The model under review builds one solid part; all positions refer to its coordinate system, in mm. A direction names the side the tool comes from. Round coordinates to 2 decimals unless told otherwise and drop trailing zeros. Write each loop counter-clockwise with the first axis right and the second up, starting at its lowest first coordinate (ties: lowest second). Pieces come first, ordered by that corner, then holes. Notation, with made-up numbers: (37.5, 73.25) - (51.5, 73.25) arc R10 cw to (51.5, 88.25) - close; hole circle Ø1 at (14.5, -0.75). An arc over 180 degrees is marked (long way). Return JSON: item names as keys, results as strings.
from build123d import *

# Parameters (mm, degrees)
EXTRUDE_1_DEPTH     = 37.9
CUT_EXTRUDE_1_REACH = 62.967
SKETCH_4_R          = 1.5
FILLET_1_R          = 0.3
FILLET_2_R          = 1


with BuildPart() as part:
    # 草图3 → 凸台-拉伸1 (new body)
    with BuildSketch(Plane.XY):
        with BuildLine():
            Line((-1.5, 0), (-4.5, 0))
            Line((-4.5, 0), (-4.5, -9))
            Line((-4.5, -9), (-1.5, -14))
            ThreePointArc((-1.5, -14), (-2.844270073, -21.5), (-1.5, -29))
            Line((-1.5, -29), (-4.5, -34))
            Line((-4.5, -34), (-4.5, -43))
            Line((-4.5, -43), (-1.5, -43))
            Line((-1.5, -43), (-1.5, -35.1))
            Line((-1.5, -35.1), (16.275513468, -35.53351048))
            ThreePointArc((16.275513468, -35.53351048), (4.5, -21.5), (16.275513468, -7.46648952))
            Line((16.275513468, -7.46648952), (-1.5, -7.9))
            Line((-1.5, -7.9), (-1.5, 0))
        make_face()
    extrude(amount=EXTRUDE_1_DEPTH)

    # 草图4 → 切除-拉伸1 (cut, up to next)
    with BuildSketch(Plane.ZY.offset(4.5), mode=Mode.PRIVATE) as cut_extrude_1_sk1:
        with Locations(Location((3, -40.7, 0), (0, 0, 270))):
            Circle(SKETCH_4_R)
    cut_extrude_1_tool1 = extrude(cut_extrude_1_sk1.sketch, amount=-CUT_EXTRUDE_1_REACH, mode=Mode.PRIVATE) & part.part
    # 草图4 → 切除-拉伸1 (cut, up to next)
    with BuildSketch(Plane.ZY.offset(4.5), mode=Mode.PRIVATE) as cut_extrude_1_sk2:
        with Locations(Location((34.9, -40.7, 0), (0, 0, 270))):
            Circle(SKETCH_4_R)
    cut_extrude_1_tool2 = extrude(cut_extrude_1_sk2.sketch, amount=-CUT_EXTRUDE_1_REACH, mode=Mode.PRIVATE) & part.part
    # 草图4 → 切除-拉伸1 (cut, up to next)
    with BuildSketch(Plane.ZY.offset(4.5), mode=Mode.PRIVATE) as cut_extrude_1_sk3:
        with Locations(Location((3, -2.3, 0), (0, 0, 270))):
            Circle(SKETCH_4_R)
    cut_extrude_1_tool3 = extrude(cut_extrude_1_sk3.sketch, amount=-CUT_EXTRUDE_1_REACH, mode=Mode.PRIVATE) & part.part
    # 草图4 → 切除-拉伸1 (cut, up to next)
    with BuildSketch(Plane.ZY.offset(4.5), mode=Mode.PRIVATE) as cut_extrude_1_sk4:
        with Locations(Location((34.9, -2.3, 0), (0, 0, 270))):
            Circle(SKETCH_4_R)
    cut_extrude_1_tool4 = extrude(cut_extrude_1_sk4.sketch, amount=-CUT_EXTRUDE_1_REACH, mode=Mode.PRIVATE) & part.part
    add(cut_extrude_1_tool1.solids().sort_by_distance((-4.5, -40.7, 3))[0], mode=Mode.SUBTRACT)
    add(cut_extrude_1_tool2.solids().sort_by_distance((-4.5, -40.7, 34.9))[0], mode=Mode.SUBTRACT)
    add(cut_extrude_1_tool3.solids().sort_by_distance((-4.5, -2.3, 3))[0], mode=Mode.SUBTRACT)
    add(cut_extrude_1_tool4.solids().sort_by_distance((-4.5, -2.3, 34.9))[0], mode=Mode.SUBTRACT)

    # 圆角1
    fillet_1_edges = [part.edges().sort_by_distance(p)[0] for p in [
        (16.275513468, -35.53351048, 18.95),
        (16.275513468, -7.46648952, 18.95),
    ]]
    fillet(fillet_1_edges, radius=FILLET_1_R)

    # 圆角2
    fillet_2_edges = [part.edges().sort_by_distance(p)[0] for p in [
        (-3, -43, 0),
        (-3, 0, 0),
        (-3, 0, 37.9),
        (-1.5, -35.1, 18.95),
        (-4.5, -34, 18.95),
        (-1.5, -29, 18.95),
        (-1.5, -14, 18.95),
        (-4.5, -9, 18.95),
        (-1.5, -7.9, 18.95),
        (-3, -43, 37.9),
    ]]
    fillet(fillet_2_edges, radius=FILLET_2_R)


solid = part.part
(1) Clearance check with flat-ended pins moving along their axes: pin 1 Ø3.5 at (y, z) = (-40, 14.5) entering from +X; pin 2 Ø1.5 at (y, z) = (-19, 5) entering from +X; pin 3 Ø8 at (y, z) = (-28.5, 14.5) entering from -X. State where each tip first meets the part, or that it passes through.
Filled in:
{"pin 1": "stops at x = -1.5", "pin 2": "stops at x = 4.88", "pin 3": "stops at x = -3.6"}
(2) Add section D-D (z = 22). Write out the cut boundary in (x, y).
Filled in:
{"outline": "(-4.5, -43) - (-1.5, -43) - (-1.5, -36.12) arc R1 cw to (-0.48, -35.12) - (13.77, -35.47) arc R0.3 ccw to (13.88, -34.89) arc R14.25 cw to (13.88, -8.11) arc R0.3 ccw to (13.77, -7.53) - (-0.48, -7.88) arc R1 cw to (-1.5, -6.88) - (-1.5, 0) - (-4.5, 0) - (-4.5, -8.72) arc R1 ccw to (-4.36, -9.24) - (-1.74, -13.59) arc R1 cw to (-1.66, -14.44) arc R21.59 ccw to (-1.66, -28.56) arc R1 cw to (-1.74, -29.41) - (-4.36, -33.76) arc R1 ccw to (-4.5, -34.28) - close"}
(3) For faces 1 (the cylindrical face through (-1.19, -7.6, 19.22)), 2 (the flat face through (-1.5, -3, 19)), 3 (the flat face through (-3.03, -31.55, 18.68)), list the 3-axis set-ups (+Z, -Z, +X, -X, +Y, -Y) from which the entire face can be reached by the end or side of a thin tool; tool diameter is ignored.
Filled in:
{"face 1": "+Z, -Z, +Y", "face 2": "+Z, -Z, +X, +Y", "face 3": "+Z, -Z, -X"}
(4) Wall thickness on line 1 (Z direction, x = -2.2, y = -40.7); line 2 (Y direction, x = 10.75, z = 21); line 3 (X direction, y = -37, z = 13.5): over which ranges is each line inside the solid? List them lowest first.
Filled in:
{"line 1": "z = 0 to 1.5, 4.5 to 33.4, 36.4 to 37.9", "line 2": "y = -35.4 to -33.29, -9.71 to -7.6", "line 3": "x = -4.5 to -1.5"}
(5) Mouldability with a two-part tool opening along Z and no side actions: class faces 4 (the cylindrical face through (-3, -39.5, 2.1)), 5 (the flat face through (-4.5, -39, 19)), 6 (the cylindrical face through (-3, -39.5, 34)), 7 (the flat face through (3, -26, 0)) as released by +Z, released by -Z, zero draft, split by the parting line, or undercut.
Filled in:
{"face 4": "undercut", "face 5": "zero draft", "face 6": "undercut", "face 7": "released by -Z"}
(6) Add section A-A (z = 34.9). Write out the cut boundary in (x, y), plus the area to 3 significant figures.
Filled in:
{"outline": "(-4.5, -43) - (-1.5, -43) - (-1.5, -42.2) - (-4.5, -42.2) - close; (-4.5, -39.2) - (-1.5, -39.2) - (-1.5, -36.12) arc R1 cw to (-0.48, -35.12) - (13.77, -35.47) arc R0.3 ccw to (13.88, -34.89) arc R14.25 cw to (13.88, -8.11) arc R0.3 ccw to (13.77, -7.53) - (-0.48, -7.88) arc R1 cw to (-1.5, -6.88) - (-1.5, -3.8) - (-4.5, -3.8) - (-4.5, -8.72) arc R1 ccw to (-4.36, -9.24) - (-1.74, -13.59) arc R1 cw to (-1.66, -14.44) arc R21.59 ccw to (-1.66, -28.56) arc R1 cw to (-1.74, -29.41) - (-4.36, -33.76) arc R1 ccw to (-4.5, -34.28) - close; (-4.5, -0.8) - (-1.5, -0.8) - (-1.5, 0) - (-4.5, 0) - close", "area": "306 mm2"}
(7) Add section C-C (x = 8.75). Write out the cut boundary in (y, z), plus the area to 3 significant figures.
Filled in:
{"outline": "(-35.35, 0) - (-31.65, 0) - (-31.65, 37.9) - (-35.35, 37.9) - close; (-11.35, 0) - (-7.65, 0) - (-7.65, 37.9) - (-11.35, 37.9) - close", "area": "280 mm2"}
(8) Add section B-B (y = -40.7). Write out the cut boundary in (x, z).
Filled in:
{"outline": "(-4.5, 0) - (-1.5, 0) - (-1.5, 1.5) - (-4.5, 1.5) - close; (-4.5, 4.5) - (-1.5, 4.5) - (-1.5, 33.4) - (-4.5, 33.4) - close; (-4.5, 36.4) - (-1.5, 36.4) - (-1.5, 37.9) - (-4.5, 37.9) - close"}
